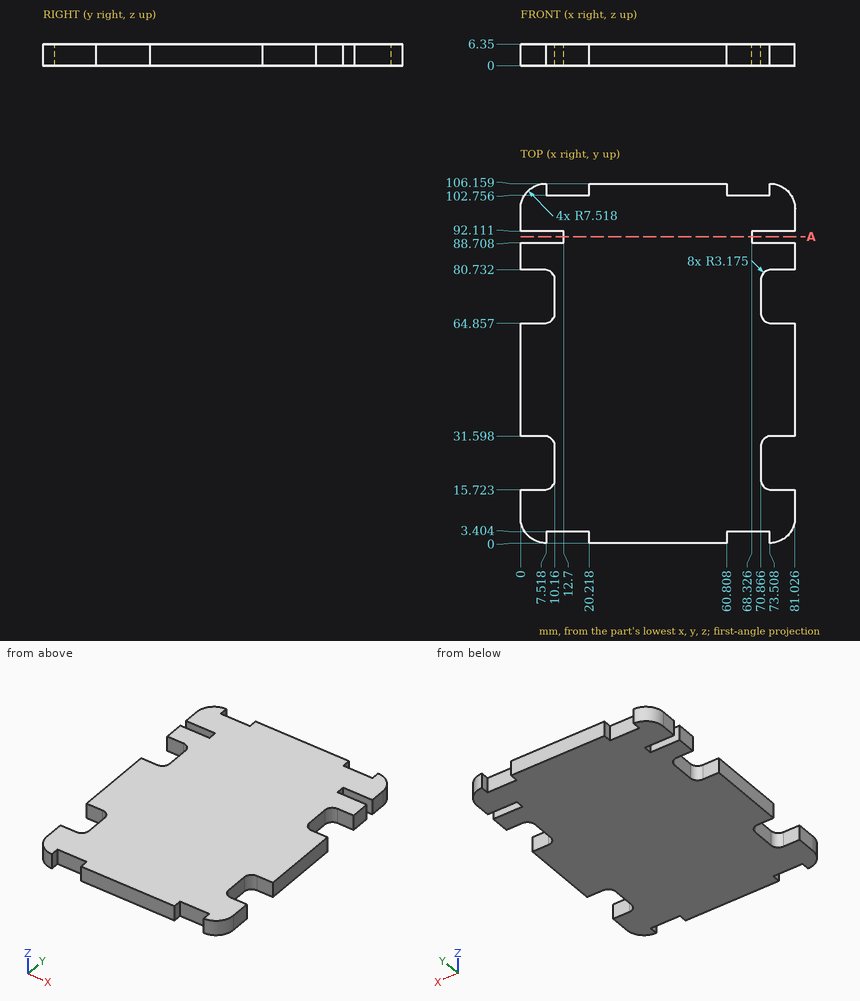
Job drawing, mm, ordinate dimensions from the low corner. One solid piece. Coordinates: 2 decimals unless noted, no trailing zeros. Order: outer loops, then holes, each group sorted by start corner. A loop starts at its lowest first (then second) coordinate and runs counter-clockwise, first axis right, second up. Notation, with made-up numbers: (68.5, 85.5) -> (82.5, 85.5) arc R32 cw to (82.5, 120.5) -> close; hole circle Ø2 at (39.5, -19). An arc over 180 degrees is marked (long way). Return JSON: item names as keys, results as strings. Group by question number.
Item 1: Flat gauge pins, fed straight in: P1, Ø2.5, axis at y = 1.5, z = 3.5, coming from the -X side (1 decimal); P2, Ø2, axis at x = 69, z = 4.5, coming from the +Y side; P3, Ø3, axis at y = 72, z = 3.5, coming from the +X side. Where does each tip first touch, or does it go through?
Item 2: Wall check: line 1 along Y through (x, z) = (77, 0.5); line 2 along Y through (x, z) = (12.5, 4.5) (1 decimal); line 3 along Y through (x, z) = (5, 4.5) (1 decimal). Give the ranges that are in metal, low to high. Write a range as [from, to].
Item 3: Saw through at A-A on y = 90.5. Write the cut outline in (x, z).
Values found:
{
 "1": {"P1": "stops at x = 1.7", "P2": "stops at y = 102.76", "P3": "stops at x = 70.87"},
 "2": {"line 1": "y = [0.86, 15.72], [31.6, 64.86], [80.73, 88.71], [92.11, 105.3]", "line 2": "y = [3.4, 88.7], [92.1, 102.8]", "line 3": "y = [0.4, 15.7], [31.6, 64.9], [80.7, 88.7], [92.1, 105.7]"},
 "3": {"outline": "(12.7, 0) -> (68.33, 0) -> (68.33, 6.35) -> (12.7, 6.35) -> close"}
}
